The model under review builds one solid part; all positions refer to its coordinate system, in mm. Give positions to 0.01 mm unless a question says otherwise; leave off trailing zeros. Loops run counter-clockwise (first coordinate to the right, second up) from the corner with the lowest first, then second, coordinate; pieces in that order, holes last. Notation, with made-up numbers: M 62,-3.5 L 112,-3.5 A30 ccw 112,35.5 Z; hole C -30,14.5 d10. An arc over 180 degrees is marked long. Put each result on its own line as item: value. Start each with the question number.
```python
from build123d import *

# Parameters (mm, degrees)
SKETCH1_R           = 12.3
BOSS_EXTRUDE1_DEPTH = 12
SKETCH2_R           = 30
BOSS_EXTRUDE2_DEPTH = 4
SKETCH3_R           = 2.5
CUT_EXTRUDE1_DEPTH  = 5
SKETCH4_R           = 6.5
CUT_EXTRUDE2_DEPTH  = 17
CUT_EXTRUDE3_DEPTH  = 5


with BuildPart() as part:
    # Sketch1 → Boss-Extrude1 (new body)
    with BuildSketch(Plane(origin=(0, 0, 0), x_dir=(0, 1, 0), z_dir=(0, 0, 1))):
        Circle(SKETCH1_R)
    extrude(amount=BOSS_EXTRUDE1_DEPTH)

    # Sketch2 → Boss-Extrude2 (add)
    with BuildSketch(Plane.XY.offset(12)):
        Circle(SKETCH2_R)
    extrude(amount=BOSS_EXTRUDE2_DEPTH)

    # Sketch3 → Cut-Extrude1 (cut, through all)
    with BuildSketch(Plane(origin=(0, 0, 12), x_dir=(1, 0, 0), z_dir=(0, 0, -1))):
        with Locations((0, 23)):
            Circle(SKETCH3_R)
        with Locations((0, -23)):
            Circle(SKETCH3_R)
    extrude(amount=-CUT_EXTRUDE1_DEPTH, mode=Mode.SUBTRACT)

    # Sketch4 → Cut-Extrude2 (cut, through all)
    with BuildSketch(Plane(origin=(0, 0, 0), x_dir=(1, 0, 0), z_dir=(0, 0, -1))):
        Circle(SKETCH4_R)
    extrude(amount=-CUT_EXTRUDE2_DEPTH, mode=Mode.SUBTRACT)

    # Sketch5 → Cut-Extrude3 (cut, through all)
    with BuildSketch(Plane(origin=(0, 0, 12), x_dir=(1, 0, 0), z_dir=(0, 0, -1))):
        with BuildLine():
            Line((-16.583123952, -25), (-16.583123952, 25))
            ThreePointArc((-16.583123952, 25), (-30, 0), (-16.583123952, -25))
        make_face()
        with BuildLine():
            Line((16.583123952, -25), (16.583123952, 25))
            ThreePointArc((16.583123952, 25), (30, 0), (16.583123952, -25))
        make_face()
    extrude(amount=-CUT_EXTRUDE3_DEPTH, mode=Mode.SUBTRACT)


solid = part.part
```
Item 1: Consider section B-B, the plane z = 13.5. Write out the cut boundary in (x, y), plus the area to 3 significant figures.
Item 2: To check wall thickness, follow L1, parallel to X at y = 23, z = 14; L2, parallel to Z at x = -4, y = 18; L3, parallel to X at y = 3.5, z = 7. State the ranges of each line that lie inside material, in increasing order. Write a range as [from, to].
Item 3: Consider section A-A, the plane y = 23. Write out the cut boundary in (x, z).
Item 4: Consider section D-D, the plane y = 0. Write out the cut boundary in (x, z).
Item 5: Clearance check with flat-ended pins moving along their axes: pin 1 Ø1 at (x, z) = (-7, 10) entering from -Y; pin 2 Ø6 at (x, z) = (3, 3.5) entering from +Y; pin 3 Ø10 at (x, y) = (-6.5, -6.5) entering from -Z; pin 4 Ø5 at (x, z) = (6, 14) entering from +Y. State where each tip first meets the part, or that it passes through.
Item 6: Consider section C-C, the plane x = 1.5. Write out the cut boundary in (y, z).
Item 7: Draft analysis for pull direction X (two halves, no side actions). For faces 1 (the cylindrical face through (12, -2.7, 5.9)), 2 (the flat face through (11, -6, 12)), 3 (the cylindrical face through (-0.33, 20.52, 13.97)), 4 (the cylindrical face through (-0.33, -25.48, 13.97)), state which applies: +X half, -X half, draft (parallel to the pull), parting line (faces both ways), or undercut.
Report:
1. outline: M -16.58,-25 A30 ccw 16.58,-25 L 16.58,25 A30 ccw -16.58,25 Z; hole C 0,0 d13; hole C 0,-23 d5; hole C 0,23 d5
1. area: 1,710 mm²
2. L1: [-16.58, -2.5], [2.5, 16.58]
2. L2: [12, 16]
2. L3: [-11.79, -5.48], [5.48, 11.79]
3. outline: M -16.58,12 L -2.5,12 L -2.5,16 L -16.58,16 Z; M 2.5,12 L 16.58,12 L 16.58,16 L 2.5,16 Z
4. outline: M -16.58,12 L -12.3,12 L -12.3,0 L -6.5,0 L -6.5,16 L -16.58,16 Z; M 6.5,0 L 12.3,0 L 12.3,12 L 16.58,12 L 16.58,16 L 6.5,16 Z
5. pin 1: y = -10.44
5. pin 2: y = 12.3
5. pin 3: z = 0
5. pin 4: y = 29.8
6. outline: M -29.96,12 L -25,12 L -25,16 L -29.96,16 Z; M -21,12 L -12.21,12 L -12.21,0 L -6.32,0 L -6.32,16 L -21,16 Z; M 6.32,0 L 12.21,0 L 12.21,12 L 21,12 L 21,16 L 6.32,16 Z; M 25,12 L 29.96,12 L 29.96,16 L 25,16 Z
7. face 1: parting line
7. face 2: draft
7. face 3: undercut
7. face 4: undercut
